from build123d import *

# Parameters (mm, degrees)
F0_R     = 5.5
F1_DEPTH = 9
F3_DEPTH = 9
F4_R     = 7
F5_DEPTH = 9


with BuildPart() as f1:
    # F0 (on Top) → F1 (new body)
    with BuildSketch(Plane.XY):
        with BuildLine():
            Line((59, 0), (0, 0))
            Line((0, 0), (0, -24))
            ThreePointArc((0, -24), (3.807612, -33.192388), (13, -37))
            Line((13, -37), (46, -37))
            ThreePointArc((46, -37), (55.192388, -33.192388), (59, -24))
            Line((59, -24), (59, 0))
        make_face()
        with Locations((13, -24)):
            Circle(F0_R, mode=Mode.SUBTRACT)
        with Locations((46, -24)):
            Circle(F0_R, mode=Mode.SUBTRACT)
    extrude(amount=F1_DEPTH)

    # F2 (on face) → F3 (join)
    with BuildSketch(Plane(origin=(0, 0, 0), x_dir=(-1, 0, 0), z_dir=(0, 1, 0))):
        Polygon((-59, 9), (0, 9), (-60.686292, 75.313708), (-83.313708, 52.686292), (-59, 0), align=None)
    extrude(amount=-F3_DEPTH)

    # F4 (on face) → F5 (join)
    with BuildSketch(Plane(origin=(68, 0, 68), x_dir=(0, 1, 0), z_dir=(0.707107, 0, 0.707107))):
        with BuildLine():
            Line((-29, -21.656854), (0, -21.656854))
            Line((0, -21.656854), (0, 10.343146))
            Line((0, 10.343146), (-29, 10.343146))
            ThreePointArc((-29, 10.343146), (-45, -5.656854), (-29, -21.656854))
        make_face()
        with Locations((-29, -5.656854)):
            Circle(F4_R, mode=Mode.SUBTRACT)
    extrude(amount=-F5_DEPTH)


solid = f1.part
The listing builds one solid part. Answer for the finished solid, in the listing's coordinates (mm). A direction names the side the tool comes from. Give positions to 0.01 mm unless a question says otherwise; leave off trailing zeros. Loops run counter-clockwise (first coordinate to the right, second up) from the corner with the lowest first, then second, coordinate; pieces in that order, holes last.
Item 1: A tool of negligible diameter and unlimited length cuts with its end or side. For faces 5 (the flat face through (62.96, -22.82, 60.31)), 6 (the flat face through (71.327, -4.437, 26.712)), 7 (the cylindrical face through (55.091, -33.293, 4.437)), from which of +Z, -Z, +X, -X, +Y, -Y can it reach the whole face along a straight path? Write none if from no direction.
Derived:
face 5: -X, -Y
face 6: -Z, +X, +Y, -Y
face 7: -Z, +X, -Y
Item 2: Determine the mould class of faces 1 (the flat face through (29, -18, 0)), 2 (the cylindrical face through (70.758, -22.534, 58.967)), 3 (the flat face through (42, 0, 27)), 4 (the cylindrical face through (69, -45, 61)) for opening direction Y: +Y half, -Y half, draft (parallel to the pull), parting line (faces both ways), or undercut.
Derived:
face 1: draft
face 2: undercut
face 3: +Y half
face 4: -Y half
Item 3: Each of these flat-tipped pins is pushed along its axis until it touches: pin 1 Ø1.5 at (y, z) = (-26.5, 58) entering from -X; pin 2 Ø7 at (y, z) = (-14.5, 5.5) entering from +X; pin 3 Ø10 at (x, y) = (13, -24) entering from -Z; pin 4 Ø2 at (x, z) = (28.5, 40) entering from -Y. Where does it stop, or does it pass through?
Derived:
pin 1: stops at x = 74.38
pin 2: stops at x = 59
pin 3: passes through
pin 4: stops at y = -9
Item 4: Find the intervals of material crossed by line 1 along Y through (x, z) = (46, 3.25); line 2 along Y through (x, z) = (69.5, 33.5); line 3 along Y through (x, z) = (24.5, 6.5), in increasing order.
Derived:
line 1: y = -37 to -29.5, -18.5 to 0
line 2: y = -9 to 0
line 3: y = -37 to 0
Item 5: A cutting plane is placed at C-C (x = 11). Give the vertices of the cut face in (y, z).
Derived:
outline: (-36.85, 0) - (-29.12, 0) - (-29.12, 9) - (-36.85, 9) - close; (-18.88, 0) - (0, 0) - (0, 21.02) - (-9, 21.02) - (-9, 9) - (-18.88, 9) - close
Item 6: A cutting plane is placed at A-A (y = -16). Give the vertices of the cut face in (x, z).
Derived:
outline: (0, 0) - (59, 0) - (59, 9) - (0, 9) - close; (54.32, 68.95) - (76.95, 46.32) - (83.31, 52.69) - (60.69, 75.31) - close
Item 7: A cutting plane is placed at D-D (z = 13). Give the vertices of the cut face in (x, y), then the cut area to 3 significant figures.
Derived:
outline: (3.66, -9) - (65, -9) - (65, 0) - (3.66, 0) - close
area: 552 mm2
